CAD build for the part. Positions are in the model's coordinates, mm. Face numbers are marked on the shaded views. Round coordinates to 2 decimals unless told otherwise and drop trailing zeros. Loops run counter-clockwise (first coordinate to the right, second up) from the corner with the lowest first, then second, coordinate; pieces in that order, holes last. Notation, with made-up numbers: (3.25, 13.5) -> (14.25, 13.5) arc R23 cw to (14.25, 21.5) -> close; hole circle Ø5 at (-40, 55). An arc over 180 degrees is marked (long way). Answer as CSV lines item,"result".
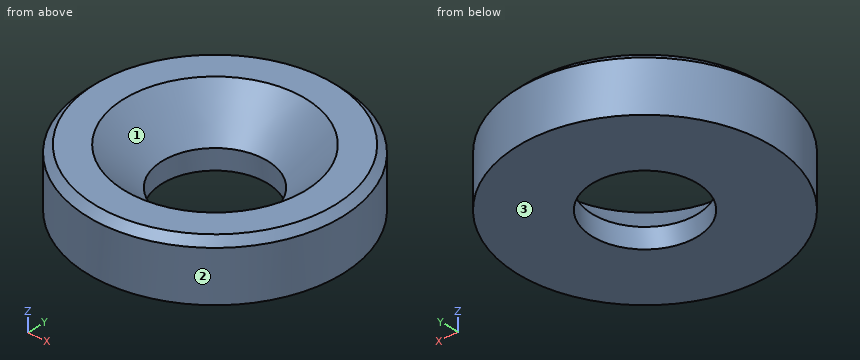
Solid Edge part; units mm, degrees
sketch "Sketch1" plane through (0, 0, 0) normal (0, 0, 1) x (1, 0, 0)
  circle A0 centre (0, 0) radius 17.5
extrude "Protrusion1" add sketch "Sketch1" along normal blind 8
hole "Hole_1" at (0, 0, 8) direction (0, 0, -1) diameter 14.5 end up to next countersink diameter 25 countersink angle 90
chamfer "Chamfer_1" distance 1 angle 45 1 edges at (-17.5, 0, 8)
Q1. Two-plate mould, pull along Y, no slides. Class the marked faces 1, 2 and 3: pulls with the +Y half, pulls with the -Y half, needs draft (parallel to the pull), parting line crosses it, or undercut.
Results:
face 1,"undercut"
face 2,"parting line crosses it"
face 3,"needs draft"
Q2. Slice it at D-D, the plane z = 5. Give the cut face in (x, y), and give its area (3 significant figures).
Results:
outline,"circle Ø35 at (0, 0); hole circle Ø19 at (0, 0)"
area,"679 mm2"
Q3. Drop flat-ended pins along their axis: pin 1 Ø1.5 at (x, z) = (-9.5, 1.5) entering from +Y; pin 2 Ø3 at (x, z) = (-1, 4.5) entering from +Y; pin 3 Ø2 at (x, z) = (4.5, 5.5) entering from +Y; pin 4 Ø1.5 at (x, z) = (10, 5.5) entering from +Y. Give the stop position or say it passes through.
Results:
pin 1,"y = 15.16"
pin 2,"y = 17.5"
pin 3,"y = 17.15"
pin 4,"y = 14.86"
Q4. Probe L1, parallel to Y at x = 0, z = 2; L2, parallel to X at y = 4, z = 3.25; L3, parallel to Z at x = 7.5, y = 8.5. List the from-to ranges inside material, lowest first. Write a range as [from, to].
Results:
L1,"[-17.5, -7.25], [7.25, 17.5]"
L2,"[-17.04, -6.64], [6.64, 17.04]"
L3,"[0, 6.84]"
Q5. Slice it at A-A, the plane x = 0. Give the cut face in (y, z), and give its area (3 significant figures).
Results:
outline,"(-17.5, 0) -> (-7.25, 0) -> (-7.25, 2.75) -> (-12.5, 8) -> (-16.5, 8) -> (-17.5, 7) -> close; (7.25, 0) -> (17.5, 0) -> (17.5, 7) -> (16.5, 8) -> (12.5, 8) -> (7.25, 2.75) -> close"
area,"135 mm2"
Q6. Slice it at C-C, the plane z = 1.5. Give the cut face in (x, y).
Results:
outline,"circle Ø35 at (0, 0); hole circle Ø14.5 at (0, 0)"
